Verification items for this drawing (mm, ordinates from the low corner). Give positions to 0.01 mm unless a question says otherwise; leave off trailing zeros. Write each loop counter-clockwise with the first axis right and the second up, starting at its lowest first coordinate (ties: lowest second). Pieces come first, ordered by that corner, then holes. Notation, with made-up numbers: (58, 61.25) -> (89, 61.25) arc R16 cw to (89, 89.25) -> close; hole circle Ø6 at (81, -36). An arc over 180 degrees is marked (long way). Write item = value, one per line.
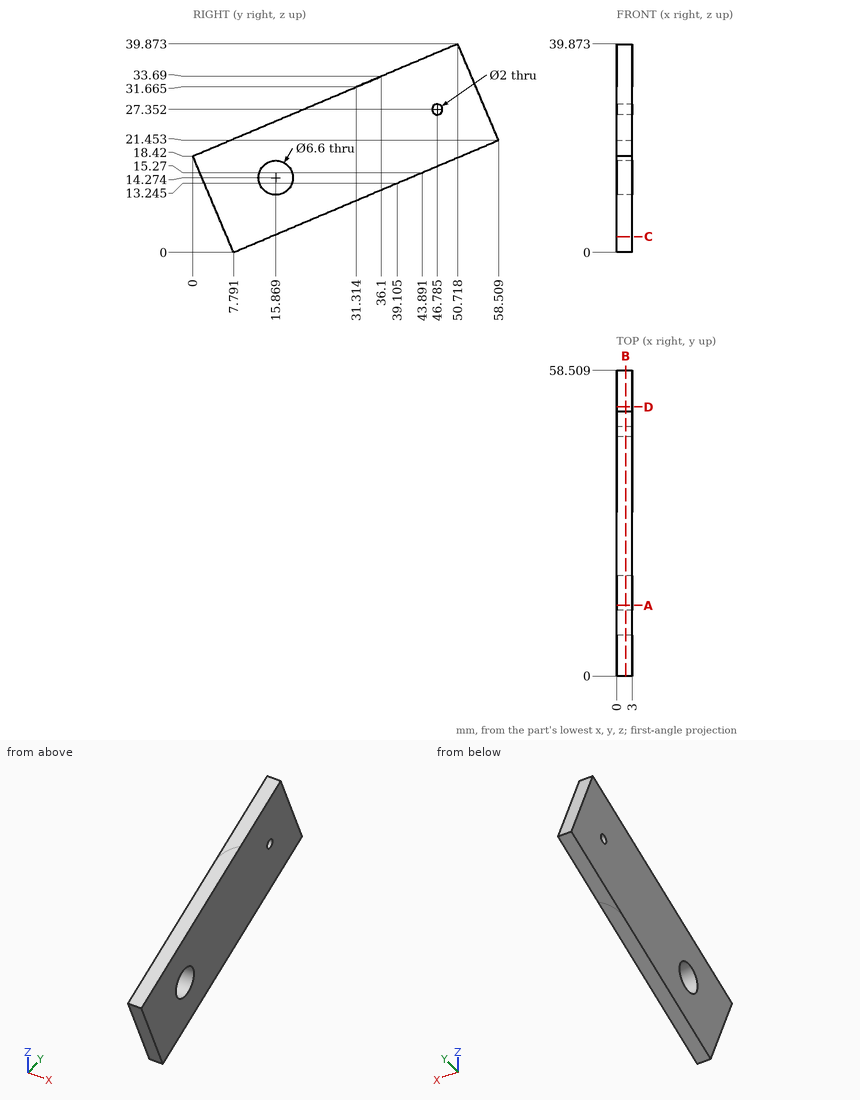
Item 1: Sectioned sample at A-A on y = 13.5. Record the cut outline in (x, z) (1 decimal).
Response values:
outline = (0, 2.4) -> (3, 2.4) -> (3, 12) -> (0, 12) -> close; (0, 16.6) -> (3, 16.6) -> (3, 24.1) -> (0, 24.1) -> close
Item 2: Go/stop test with flat-tipped pins: P1, Ø1, axis at x = 1, y = 19, coming from the +Z side; P2, Ø1, axis at x = 2.5, z = 17.5, coming from the -Y side. Record where each tip stops, or that it passes through.
Response values:
P1 = 26.67
P2 = 0.18
Item 3: Sectioned sample at B-B on x = 1.75. Record the cut outline in (y, z) (1 decimal), then the cut area to 3 significant figures.
Response values:
outline = (0, 18.4) -> (7.8, 0) -> (58.5, 21.5) -> (50.7, 39.9) -> close; hole circle Ø6.6 at (15.9, 14.3); hole circle Ø2 at (46.8, 27.4)
area = 1,060 mm^2
Item 4: Sectioned sample at D-D on y = 51.5. Record the cut outline in (x, z) (1 decimal), then the cut area to 3 significant figures.
Response values:
outline = (0, 18.5) -> (3, 18.5) -> (3, 38) -> (0, 38) -> close
area = 58.6 mm^2
Item 5: Sectioned sample at C-C on z = 3. Record the cut outline in (x, y), then the cut area to 3 significant figures.
Response values:
outline = (0, 6.52) -> (3, 6.52) -> (3, 14.88) -> (0, 14.88) -> close
area = 25.1 mm^2
Item 6: Material ranges on line 1 (Y direction, x = 0.3, z = 16) (1 decimal); line 2 (Y direction, x = 2.5, z = 13) (1 decimal); line 3 (Z direction, x = 0.3, y = 12) (1 decimal), recorded low to high.
Response values:
line_1 = 1 to 13.1, 18.7 to 45.6
line_2 = 2.3 to 12.8, 18.9 to 38.5
line_3 = 1.8 to 23.5
